Geometry: final body of the model. Coordinates: model frame, mm. Face numbers are marked on the shaded views. A direction names the side the tool comes from. Give positions to 0.01 mm unless a question says otherwise; leave off trailing zeros. Loops run counter-clockwise (first coordinate to the right, second up) from the corner with the lowest first, then second, coordinate; pieces in that order, holes last. Notation, with made-up numbers: (30.25, 42) - (43.25, 42) arc R23 cw to (43.25, 52) - close; hole circle Ø1 at (-12, 17.5). An arc over 180 degrees is marked (long way). Use one line per item in the form item = value.
Autodesk Inventor part; units mm, degrees
ref_plane "工作平面1" through (-21, -48, 24) normal (0, -0.7071, 0.7071) x (1, 0, 0)
ref_plane "YZ Plane" through (0, 0, 0) normal (1, 0, 0) x (0, 1, 0)
ref_plane "XZ Plane" through (0, 0, 0) normal (0, 1, 0) x (-1, 0, 0)
sketch "草图2" plane through (0, 0, 0) normal (0, 1, 0) x (-1, 0, 0)
  line L0 (-21, 21) -> (21, 21)
  line L1 (21, 21) -> (21, -21)
  line L2 (21, -21) -> (-21, -21)
  line L3 (-21, -21) -> (-21, 21)
  line L4 (-21, 21) -> (21, -21) construction
  line L5 (21, 21) -> (-21, -21) construction
  point P0 (0, 0)
  dimension "d3" = 42
  dimension "d4" = 42
extrude "拉伸2" add sketch "草图2" along normal blind 3
sketch "草图3" plane through (-21, 0, 21) normal (0, 0, 1) x (1, 0, 0)
  line L0 (0, 3) -> (42, 3)
  line L1 (0, 3) -> (42, 3)
  line L2 (42, 3) -> (42, -48)
  line L3 (42, -48) -> (0, -48)
  line L4 (0, -48) -> (0, 3)
  point P0 (21, 0)
  dimension "d7" = 51
extrude "拉伸3" add sketch "草图3" along normal blind 3
ref_plane "工作平面1" through (-21, -48, 24) normal (0, -0.7071, 0.7071) x (1, 0, 0)
sketch "草图7" plane through (0, 0, 0) normal (0, -1, 0) x (1, 0, 0)
  circle A0 centre (0, 0) radius 11.5
  circle A1 centre (-15.5, 15.5) radius 1.75
  circle A2 centre (-15.5, -15.5) radius 1.75
  circle A3 centre (15.5, -15.5) radius 1.75
  circle A4 centre (15.5, 15.5) radius 1.75
  dimension "d17" = 23
  dimension "d18" = 3.5
  dimension "d19" = 15.5
  dimension "d20" = 15.5
  dimension "d21" = 15.5
  dimension "d22" = 15.5
extrude "拉伸6" cut sketch "草图7" against normal blind 3
sketch "草图9" plane through (-21, 0, 24) normal (0, 0, 1) x (1, 0, 0)
  line L0 (0, 0) -> (0, -48)
  line L1 (42, -48) -> (42, 0)
  line L2 (0, -28) -> (42, -28)
  line L3 (42, -28) -> (42, -25)
  line L4 (42, -25) -> (0, -25)
  line L5 (0, -25) -> (0, -28)
  line L6 (0, -48) -> (42, -48)
  point P0 (21, 0)
  dimension "d32" = 3
  dimension "d33" = 20
extrude "拉伸8" add sketch "草图9" along normal blind 20 contours L4 L1 L2 L0
sketch "草图10" plane through (-21, 0, 24) normal (0, 0, 1) x (1, 0, 0)
  line L0 (42, -28) -> (0, -28)
  line L1 (0, -28) -> (0, -48)
  line L2 (0, -48) -> (42, -48)
  line L3 (42, -48) -> (42, -28)
  point P0 (21, 0)
extrude "拉伸9" cut sketch "草图10" against normal blind 20
sketch "草图11" plane through (-21, -48, 24) normal (0, -0.7071, 0.7071) x (1, 0, 0)
  line L0 (0, 28.2843) -> (42, 28.2843)
  line L1 (0, 28.2843) -> (42, 28.2843)
  line L2 (42, 28.2843) -> (42, 78.2843)
  line L3 (42, 78.2843) -> (0, 78.2843)
  line L4 (0, 78.2843) -> (0, 28.2843)
  point P0 (21, 16.9706)
  dimension "d38" = 42
  dimension "d39" = 50
extrude "拉伸10" add sketch "草图11" against normal blind 3
sketch "草图12" plane through (-21, -48, 24) normal (0, -0.7071, 0.7071) x (1, 0, 0)
  line L0 (0, 28.2843) -> (42, 28.2843) construction
  line L1 (21, 28.2843) -> (21, 78.2843) construction
  line L2 (0, 78.2843) -> (42, 78.2843) construction
  circle A0 centre (31, 43.2843) radius 3
  circle A1 centre (31, 68.2843) radius 3
  circle A2 centre (11, 43.2843) radius 3
  circle A3 centre (11, 68.2843) radius 3
  point P0 (21, 16.9706)
  dimension "d42" = 6
  dimension "d43" = 10
  dimension "d44" = 15
  dimension "d45" = 25
extrude "拉伸11" cut sketch "草图12" against normal blind 3
properties part number "电机座1"
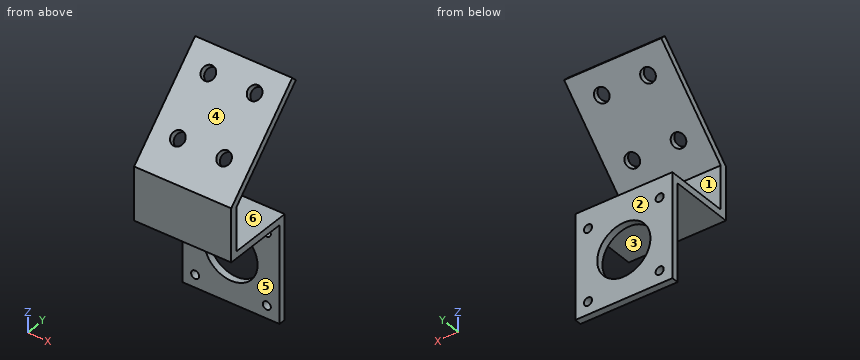
(1) Cut plane D-D (x = 15.5). Give the number of separate pieces and of enclosed holes in the cut face, plus the area to 3 significant figures.
Solution:
separate_pieces = 3
enclosed_holes = 0
area = 404 mm2
(2) Cut plane C-C (z = -15.5). Return the cut outline in (x, y).
Solution:
outline = (-21, 0) - (-17.25, 0) - (-17.25, 3) - (-21, 3) - close; (-13.75, 0) - (13.75, 0) - (13.75, 3) - (-13.75, 3) - close; (17.25, 0) - (21, 0) - (21, 3) - (17.25, 3) - close
(3) Cut plane A-A (z = 0). Return the cut outline in (x, y), plus the area to 3 significant figures.
Solution:
outline = (-21, 0) - (-11.5, 0) - (-11.5, 3) - (-21, 3) - close; (11.5, 0) - (21, 0) - (21, 3) - (11.5, 3) - close
area = 57.0 mm2
(4) Material intervals for L1, parallel to X at y = 2, z = 15; L2, parallel to Z at x = -15.5, y = 1.3; L3, parallel to Z at x = 15.5, y = 2.05, sorted ascending. Write a range as from..to.
Solution:
L1 = -21..-17.18, -13.82..13.82, 17.18..21
L2 = -21..-17.25, -13.75..13.75, 17.25..24, 69.06..73.3
L3 = -21..-17.25, -13.75..13.75, 17.25..24, 69.81..74.05
(5) Pin query (flat end, axial travel): P1, Ø6, axis at x = 15, z = 32.5, coming from the +Y side; P2, Ø2, axis at x = 15.5, z = 15.5, coming from the -Y side; P3, Ø5, axis at x = -2.5, y = -16.5, coming from the -Z side; P4, Ø4.5, axis at x = -15.5, z = 15.5, coming from the +Y side. Return the tip coordinate at first contact, or that it passes through.
Solution:
P1 = -25
P2 = through
P3 = 21
P4 = 3
(6) Pull-direction query (Z, two-part tool) for the marked faces 1, 2 and 3; classes: released by +Z, released by -Z, zero draft, split by the parting line, or undercut.
Solution:
face_1 = undercut
face_2 = zero draft
face_3 = released by -Z
(7) Access query for the marked faces 4, 5 and 6. Directions: +Z, -Z, +X, -X, +Y, -Y. A direction counts if a zero-diameter tool reaches every point of the face in a straight line with its end or side. Return the directions, or none.
Solution:
face_4 = +Z, +X, -X, -Y
face_5 = -Z, +X, -X, -Y
face_6 = +X, -X, +Y
